```python
from build123d import *

# Parameters (mm, degrees)
F0_R          = 20.6375
F1_DEPTH      = 1
F1_DEPTH_BACK = 1
F3_DEPTH      = 5.35
F5_DEPTH      = 5.35


with BuildPart() as f1:
    # F0 (on Top) → F1 (new body, two sides)
    with BuildSketch(Plane.XY) as f1_sk:
        Circle(F0_R)
    extrude(amount=F1_DEPTH)
    extrude(f1_sk.sketch, amount=-F1_DEPTH_BACK)

    # F2 (on face) → F3 (join)
    with BuildSketch(Plane.XY.offset(1)):
        with BuildLine():
            Line((-10.0775, 18.009731), (-10.0775, -18.009731))
            ThreePointArc((-10.0775, -18.009731), (-8.214189, -18.93234), (-6.2675, -19.662778))
            Line((-6.2675, -19.662778), (-6.2675, 19.662778))
            ThreePointArc((-6.2675, 19.662778), (-8.214189, 18.93234), (-10.0775, 18.009731))
        make_face()
        with BuildLine():
            Line((6.2675, 19.662778), (6.2675, -19.662778))
            ThreePointArc((6.2675, -19.662778), (8.214189, -18.93234), (10.0775, -18.009731))
            Line((10.0775, -18.009731), (10.0775, 18.009731))
            ThreePointArc((10.0775, 18.009731), (8.214189, 18.93234), (6.2675, 19.662778))
        make_face()
    extrude(amount=F3_DEPTH)

    # F4 (on face) → F5 (join)
    with BuildSketch(Plane(origin=(0, 0, -1), x_dir=(1, 0, 0), z_dir=(0, 0, -1))):
        with BuildLine():
            Line((18.009731, 10.0775), (-18.009731, 10.0775))
            ThreePointArc((-18.009731, 10.0775), (-18.93234, 8.214189), (-19.662778, 6.2675))
            Line((-19.662778, 6.2675), (19.662778, 6.2675))
            ThreePointArc((19.662778, 6.2675), (18.93234, 8.214189), (18.009731, 10.0775))
        make_face()
        with BuildLine():
            Line((19.662778, -6.2675), (-19.662778, -6.2675))
            ThreePointArc((-19.662778, -6.2675), (-18.93234, -8.214189), (-18.009731, -10.0775))
            Line((-18.009731, -10.0775), (18.009731, -10.0775))
            ThreePointArc((18.009731, -10.0775), (18.93234, -8.214189), (19.662778, -6.2675))
        make_face()
    extrude(amount=F5_DEPTH)


solid = f1.part
```
Design review of the part built by this model. Coordinates are the model's own, in mm. A direction names the side the tool comes from. Coordinates: 2 decimals unless noted, no trailing zeros. Loops run counter-clockwise (first coordinate to the right, second up) from the corner with the lowest first, then second, coordinate; pieces in that order, holes last. Notation, with made-up numbers: M -8.75,25.5 L -0.75,25.5 A17 cw -0.75,37.5 Z; hole C 0,-33.75 d11. An arc over 180 degrees is marked long. One line per question, with ' | ' between items.
(1) For pin 1 Ø6 at (y, z) = (13.5, 3.5) entering from +X; pin 2 Ø4 at (x, z) = (14.5, 0) entering from -Y; pin 3 Ø2 at (y, z) = (14.5, -3.5) entering from -X; pin 4 Ø2 at (x, z) = (9.5, -5) entering from +Y, all flat-tipped, find the tip position at first contact; note any pin that passes through.
Filled in:
pin 1: stops at x = 16.9 | pin 2: stops at y = -16.42 | pin 3: passes through | pin 4: stops at y = 10.08
(2) Wall thickness on probe 1 along Y at (x, z) = (17, -4.25); probe 2 along Z at (x, y) = (6, 16): over which ranges is each line inside the solid? List them lowest first.
Filled in:
probe 1: y = -10.08 to -6.27, 6.27 to 10.08 | probe 2: z = -1 to 1
(3) Machinability: for faces 5 (the face through (14, 0, 1)), 6 (the face through (0, 14, -1)), 7 (the face through (-14, 0, 1)), 8 (the face through (-6.268, 0, 4)), which of the approach directions +Z, -Z, +X, -X, +Y, -Y give a long, thin tool a straight path to every point of the face, cutting with its end or side? Answer none if there is none.
Filled in:
face 5: +Z, +X, +Y, -Y | face 6: -Z, +X, -X, +Y | face 7: +Z, -X, +Y, -Y | face 8: +Z, +Y, -Y
(4) We need section C-C (x = 0). Give the boundary of the cut face in (y, z), and give its area (3 significant figures).
Filled in:
outline: M -20.64,-1 L -10.08,-1 L -10.08,-6.35 L -6.27,-6.35 L -6.27,-1 L 6.27,-1 L 6.27,-6.35 L 10.08,-6.35 L 10.08,-1 L 20.64,-1 L 20.64,1 L -20.64,1 Z | area: 123 mm^2
(5) We need section B-B (y = 0). Give the boundary of the cut face in (x, z).
Filled in:
outline: M -20.64,-1 L 20.64,-1 L 20.64,1 L 10.08,1 L 10.08,6.35 L 6.27,6.35 L 6.27,1 L -6.27,1 L -6.27,6.35 L -10.08,6.35 L -10.08,1 L -20.64,1 Z
(6) We need section D-D (y = -7.5). Give the boundary of the cut face in (x, z).
Filled in:
outline: M -19.23,-6.35 L 19.23,-6.35 L 19.23,1 L 10.08,1 L 10.08,6.35 L 6.27,6.35 L 6.27,1 L -6.27,1 L -6.27,6.35 L -10.08,6.35 L -10.08,1 L -19.23,1 Z
(7) We need section A-A (z = -1.75). Give the boundary of the cut face in (x, y), and give its area (3 significant figures).
Filled in:
outline: M -19.66,-6.27 A20.64 ccw -18.01,-10.08 L 18.01,-10.08 A20.64 ccw 19.66,-6.27 Z; M -19.66,6.27 L 19.66,6.27 A20.64 ccw 18.01,10.08 L -18.01,10.08 A20.64 ccw Z | area: 288 mm^2
(8) Draft analysis for pull direction Y (two halves, no side actions). For faces 1 (the face through (18.944, -8.187, -3.638)), 2 (the face through (0, 0, -1)), 3 (the face through (0, 8, -6.35)), 4 (the face through (0, -6.268, -4)), state which applies: released by +Y, released by -Y, zero draft, split by the parting line, or undercut.
Filled in:
face 1: released by -Y | face 2: undercut | face 3: zero draft | face 4: undercut
